Answer from the drawing. Dimensions are ordinates in mm from the lowest x, y and z of the part. A direction names the side the tool comes from. Round coordinates to 2 decimals unless told otherwise and drop trailing zeros. Order: outer loops, then holes, each group sorted by start corner. A loop starts at its lowest first (then second) coordinate and runs counter-clockwise, first axis right, second up. Notation, with made-up numbers: (-30.75, -5) - (-1.75, -5) arc R15 cw to (-1.75, 20) - close; hole circle Ø4 at (-19.5, 6.5). An arc over 180 degrees is marked (long way). One line per question, with ' | ' between items. Start each with the question number.
1) A flat-ended cylindrical pin translates along its axis: pin 1 (5 mm diameter, centred on x = 219, z = 143, fed in from -Y). Find the tip coordinate at first contact, or state that the pin passes through.
2) The part is cut by section D-D, the plane x = 243.5. Give the vertices of the cut face in (y, z).
3) The part is cut by section B-B, the plane y = 242.5. Give the vertices of the cut face in (x, z), plus the area to 3 significant figures.
4) The part is cut by section A-A, the plane z = 382.5. Give the vertices of the cut face in (x, y).
5) For the marked faces 1 and 2, determine the directions among +Z, -Z, +X, -X, +Y, -Y from which every point of the face is accessible in a straight line to the end or side of a thin tool.
6) Straight lines are drawn through the part: line 1 (X direction, y = 318.5, z = 129); line 2 (Z direction, x = 75, y = 271); line 3 (Z direction, x = 35, y = 28). For each, find the intervals that lie inside material, in ascending order. Write a range as from..to.
7) The mould has two halves that part along Z. Classify the marked faces 3, 4 and 5: pulls with the +Z half, pulls with the -Z half, needs draft (parallel to the pull), parting line crosses it, or undercut.
8) The part is cut by section C-C, the plane z = 30. Give the vertices of the cut face in (x, y), plus the area to 3 significant figures.
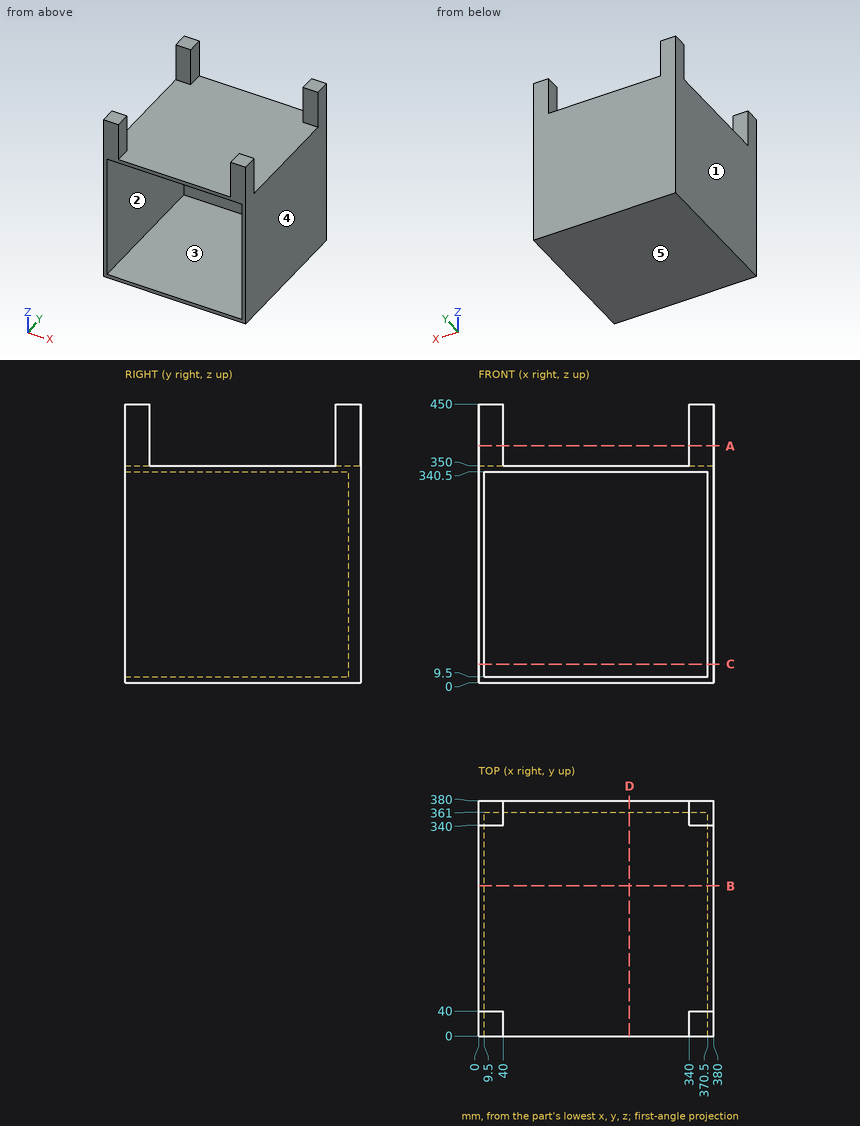
Values:
1) pin 1: stops at y = 361
2) outline: (0, 0) - (380, 0) - (380, 350) - (0, 350) - (0, 340.5) - (361, 340.5) - (361, 9.5) - (0, 9.5) - close
3) outline: (0, 0) - (380, 0) - (380, 350) - (0, 350) - close; hole (9.5, 9.5) - (370.5, 9.5) - (370.5, 340.5) - (9.5, 340.5) - close | area: 13,500 mm^2
4) outline: (0, 0) - (40, 0) - (40, 40) - (0, 40) - close; (0, 340) - (40, 340) - (40, 380) - (0, 380) - close; (340, 0) - (380, 0) - (380, 40) - (340, 40) - close; (340, 340) - (380, 340) - (380, 380) - (340, 380) - close
5) face 1: +Z, -Z, -X, +Y, -Y | face 2: -Y
6) line 1: x = 0..9.5, 370.5..380 | line 2: z = 0..9.5, 340.5..350 | line 3: z = 0..9.5, 340.5..450
7) face 3: undercut | face 4: needs draft | face 5: pulls with the -Z half
8) outline: (0, 0) - (9.5, 0) - (9.5, 361) - (370.5, 361) - (370.5, 0) - (380, 0) - (380, 380) - (0, 380) - close | area: 14,100 mm^2
